from build123d import *

# Parameters (mm, degrees)
CROQUIS1_R                 = 16
SALIENTE_EXTRUIR1_DEPTH    = 8
CORTAR_EXTRUIR2_DEPTH      = 10
CORTAR_EXTRUIR4_DEPTH      = 5
CORTAR_EXTRUIR4_DEPTH_BACK = 10
CORTAR_EXTRUIR4_START      = -8
CROQUIS5_R                 = 1.75
SALIENTE_EXTRUIR2_DEPTH    = 9
CROQUIS6_6_R               = 1
CORTAR_EXTRUIR8_DEPTH      = 10
CROQUIS10_3_R              = 6.75
CORTAR_EXTRUIR10_DEPTH     = 2
CROQUIS13_R                = 0.375
CORTAR_EXTRUIR11_DEPTH     = 22


with BuildPart() as part:
    # Croquis1 → Saliente-Extruir1 (new body)
    with BuildSketch(Plane(origin=(0, 0, 0), x_dir=(1, 0, 0), z_dir=(0, 1, 0))):
        with Locations(Location((0, 0, 0), (0, 0, 270))):
            Circle(CROQUIS1_R)
    extrude(amount=SALIENTE_EXTRUIR1_DEPTH)

    # Croquis2 → Cortar-Extruir2 (cut)
    with BuildSketch(Plane(origin=(0, 0, 0), x_dir=(-1, 0, 0), z_dir=(0, -1, 0))):
        with BuildLine():
            ThreePointArc((-6.5, -14.620191518), (0, -16), (6.5, -14.620191517))
            Line((6.5, -14.620191517), (6.5, -10.035533906))
            Line((6.5, -10.035533906), (4.964466094, -8.5))
            Line((4.964466094, -8.5), (-4.964466094, -8.5))
            Line((-4.964466094, -8.5), (-6.5, -10.035533906))
            Line((-6.5, -10.035533906), (-6.5, -14.620191517))
        make_face()
        with BuildLine():
            Line((-4.964466094, 8.5), (4.964466094, 8.5))
            Line((4.964466094, 8.5), (6.5, 10.035533906))
            Line((6.5, 10.035533906), (6.5, 14.620191517))
            ThreePointArc((6.5, 14.620191518), (0, 16.000000001), (-6.5, 14.620191518))
            Line((-6.5, 14.620191517), (-6.5, 10.035533906))
            Line((-6.5, 10.035533906), (-4.964466094, 8.5))
        make_face()
        with BuildLine():
            Line((10.035533906, -6.5), (14.620191517, -6.5))
            ThreePointArc((14.620191515, -6.499999999), (15.651246979, -3.322418977), (15.999999994, 0))
            ThreePointArc((16, 0), (15.651246984, 3.322418978), (14.620191517, 6.5))
            Line((14.620191517, 6.5), (10.035533906, 6.5))
            Line((10.035533906, 6.5), (8.5, 4.964466094))
            Line((8.5, 4.964466094), (8.5, -4.964466094))
            Line((8.5, -4.964466094), (10.035533906, -6.5))
        make_face()
        with BuildLine():
            ThreePointArc((-14.620191518, 6.5), (-16.000000001, 0), (-14.620191518, -6.5))
            Line((-14.620191517, -6.5), (-10.035533906, -6.5))
            Line((-10.035533906, -6.5), (-8.5, -4.964466094))
            Line((-8.5, -4.964466094), (-8.5, 4.964466094))
            Line((-8.5, 4.964466094), (-10.035533906, 6.5))
            Line((-10.035533906, 6.5), (-14.620191517, 6.5))
        make_face()
    extrude(amount=-CORTAR_EXTRUIR2_DEPTH, mode=Mode.SUBTRACT)

    # Croquis4 → Cortar-Extruir4 (cut, two sides: drawn at the far end of the back side and taken through both)
    with BuildSketch(Plane.XZ.offset(CORTAR_EXTRUIR4_START - CORTAR_EXTRUIR4_DEPTH_BACK)):
        Polygon((-6.5, 16.599431938), (-6.5, 6.5), (-19.32076002, 6.5), (-19.32076002, -6.5), (-6.5, -6.5), (-6.5, -17.296221808), (6.5, -17.296221808), (6.5, -6.5), (20.964302933, -6.5), (20.964302933, 6.5), (6.5, 6.5), (6.5, 16.599431938), align=None)
    extrude(amount=CORTAR_EXTRUIR4_DEPTH + CORTAR_EXTRUIR4_DEPTH_BACK, mode=Mode.SUBTRACT)

    # Croquis5 → Saliente-Extruir2 (add)
    with BuildSketch(Plane(origin=(0, 3, 0), x_dir=(1, 0, 0), z_dir=(0, 1, 0))):
        with Locations(Location((0, 0, 0), (0, 0, 270))):
            Circle(CROQUIS5_R)
    extrude(amount=SALIENTE_EXTRUIR2_DEPTH)

    # Croquis6<6> → Cortar-Extruir8 (cut)
    with BuildSketch(Plane(origin=(0, 8, 0), x_dir=(1, 0, 0), z_dir=(0, 1, 0))):
        with Locations(Location((-9.298454173, 9.298454173, 0), (0, 0, 270))):
            Circle(CROQUIS6_6_R)
        with Locations(Location((9.298454173, 9.298454173, 0), (0, 0, 270))):
            Circle(CROQUIS6_6_R)
        with Locations(Location((9.298454173, -9.298454173, 0), (0, 0, 270))):
            Circle(CROQUIS6_6_R)
        with Locations(Location((-9.298454173, -9.298454173, 0), (0, 0, 270))):
            Circle(CROQUIS6_6_R)
    extrude(amount=-CORTAR_EXTRUIR8_DEPTH, mode=Mode.SUBTRACT)

    # Croquis10<3> → Cortar-Extruir10 (cut)
    with BuildSketch(Plane.XZ):
        with Locations(Location((0, 0, 0), (0, 0, 270))):
            Circle(CROQUIS10_3_R)
    extrude(amount=-CORTAR_EXTRUIR10_DEPTH, mode=Mode.SUBTRACT)

    # Croquis13 → Cortar-Extruir11 (cut)
    with BuildSketch(Plane.XZ):
        with Locations(Location((0, 0, 0), (0, 0, 270))):
            Circle(CROQUIS13_R)
    extrude(amount=-CORTAR_EXTRUIR11_DEPTH, mode=Mode.SUBTRACT)


solid = part.part
The listing builds one solid part. Answer for the finished solid, in the listing's coordinates (mm). A direction names the side the tool comes from. Round coordinates to 2 decimals unless told otherwise and drop trailing zeros. Order: outer loops, then holes, each group sorted by start corner. A loop starts at its lowest first (then second) coordinate and runs counter-clockwise, first axis right, second up. Notation, with made-up numbers: (70, 66) - (105, 66) arc R13 cw to (105, 90) - close; hole circle Ø2 at (40, -2). An arc over 180 degrees is marked (long way). Write item = value, one per line. Start each with the question number.
1) Section D-D, the plane x = 4.5 is taken. Write down the section's boundary in (y, z), plus the area to 3 significant figures.
2) Given pin 1 (1.5 mm diameter, centred on y = 7.5, z = 7.5, fed in from -X); pin 2 (3.5 mm diameter, centred on x = -0.5, y = 1.5, fed in from +Z); pin 3 (4 mm diameter, centred on x = -1, y = 1.5, fed in from -Z); pin 4 (1.5 mm diameter, centred on x = 3, y = 10, fed in from -Z), each flat-ended and moving along its own axis, determine where each tip first touches the part or whether it passes through.
3) For a pull along X with two mould halves and no side action, classify faces 4 (the flat face through (8.5, 1, 0)), 5 (the flat face through (0, 1, 8.5)), 6 (the flat face through (-11, 8, 10)), 7 (the flat face through (-9.257, 1.479, 5.721)) as released by +X, released by -X, zero draft, split by the parting line, or undercut.
4) Straight lines are drawn through the part: L1, parallel to Z at x = -9.5, y = 2; L2, parallel to Z at x = -5.5, y = 1.75; L3, parallel to Z at x = 10, y = 6.5. For each, find the intervals that lie inside material, in ascending order.
5) Section C-C, the plane x = 0 is taken. Write down the section's boundary in (y, z) (3 decimals).
6) For faces 1 (the flat face through (9.257, 1.479, -5.721)), 2 (the flat face through (-5.743, 1.479, 9.279)), 3 (the cylindrical face through (-1.71, 7.44, -0.38)), determine the directions among +Z, -Z, +X, -X, +Y, -Y from which every point of the face is accessible in a straight line to the end or side of a thin tool.
7) Section B-B, the plane y = 4.5 is taken. Count the separate pieces of the cut face and the enclosed holes in it, plus the area to 3 significant figures.
8) Section A-A, the plane z = 0 is taken. Write down the section's boundary in (x, y) (3 decimals), plus the area to 3 significant figures.
Results list:
q1.outline = (0, -8.5) - (3, -8.5) - (3, 8.5) - (0, 8.5) - (0, 5.03) - (2, 5.03) - (2, -5.03) - (0, -5.03) - close
q1.area = 30.9 mm^2
q2.pin_1 = -14.51
q2.pin_2 = 8.5
q2.pin_3 = -8.5
q2.pin_4 = through
q3.face_4 = released by +X
q3.face_5 = undercut
q3.face_6 = zero draft
q3.face_7 = released by -X
q4.L1 = -12.87 to -10.28, -8.32 to -5.96, 5.96 to 8.32, 10.28 to 12.87
q4.L2 = -9.04 to -3.91, 3.91 to 9.04
q4.L3 = -12.49 to -10.01, -8.59 to -6.5, 6.5 to 8.59, 10.01 to 12.49
q5.outline = (0, -8.5) - (3, -8.5) - (3, -1.75) - (12, -1.75) - (12, -0.375) - (2, -0.375) - (2, -6.75) - (0, -6.75) - close; (0, 6.75) - (2, 6.75) - (2, 0.375) - (12, 0.375) - (12, 1.75) - (3, 1.75) - (3, 8.5) - (0, 8.5) - close
q6.face_1 = +X, +Y, -Y
q6.face_2 = +Z, +Y, -Y
q6.face_3 = +Y
q7.separate_pieces = 5
q7.enclosed_holes = 5
q7.area = 161 mm^2
q8.outline = (-8.5, 0) - (-6.75, 0) - (-6.75, 2) - (-0.375, 2) - (-0.375, 12) - (-1.75, 12) - (-1.75, 3) - (-8.5, 3) - close; (0.375, 2) - (6.75, 2) - (6.75, 0) - (8.5, 0) - (8.5, 3) - (1.75, 3) - (1.75, 12) - (0.375, 12) - close
q8.area = 48.0 mm^2
